The listing builds one solid part. Answer for the finished solid, in the listing's coordinates (mm). Face numbers are marked on the shaded views. A direction names the side the tool comes from. Give positions to 0.01 mm unless a question says otherwise; leave off trailing zeros. Write each loop counter-clockwise with the first axis right and the second up, starting at its lowest first coordinate (ties: lowest second). Pieces come first, ordered by that corner, then holes. Notation, with made-up numbers: (5, -7) -> (36, -7) arc R22 cw to (36, 23) -> close; hole circle Ø4 at (-13.75, -9.5). An arc over 180 degrees is marked (long way). One line per question, with ' | ' between items.
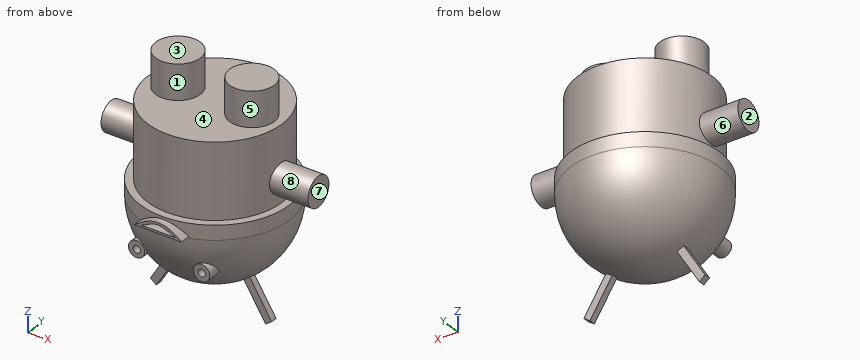
from build123d import *

# Parameters (mm, degrees)
F0_R          = 15
F3_DEPTH      = 30
F1_R          = 45
F4_DEPTH      = 50
F4_DEPTH_BACK = 6.5
F5_START      = -44
F2_R          = 50
F5_DEPTH      = 9.75
F6_R          = 10
F7_DEPTH      = 70
F8_R          = 10
F9_DEPTH      = 70
F12_R         = 5.5
F13_DEPTH     = 43.75
F14_R         = 2.5
F15_DEPTH     = 50.5
F17_DEPTH     = 4.25
F19_DEPTH     = 54.5
F21_DEPTH     = 63.5


with BuildPart() as f3:
    # F0 (on Top) → F3 (new body)
    with BuildSketch(Plane.XY):
        with Locations((-25, 0)):
            Circle(F0_R)
    extrude(amount=F3_DEPTH)



with BuildPart() as f3b:
    # F0 (on Top) → F3, piece 2 (new body)
    with BuildSketch(Plane.XY):
        with Locations((25, 0)):
            Circle(F0_R)
    extrude(amount=F3_DEPTH)


with BuildPart() as f3_1:
    add(f3.part)

    add(f3b.part)  # F4 merges F3b
    # F1 (on Top) → F4 (join, two sides)
    with BuildSketch(Plane.XY) as f4_sk:
        Circle(F1_R)
    extrude(amount=-F4_DEPTH)
    extrude(f4_sk.sketch, amount=F4_DEPTH_BACK)

    # F2 (on Top) → F5 (join)
    with BuildSketch(Plane.XY.offset(F5_START)):
        Circle(F2_R)
    extrude(amount=-F5_DEPTH)

    # F6 (on Right) → F7 (join)
    with BuildSketch(Plane.YZ):
        with Locations((0, -28)):
            Circle(F6_R)
    extrude(amount=F7_DEPTH)

    # F8 (on Right) → F9 (join)
    with BuildSketch(Plane.YZ):
        with Locations((0, -28)):
            Circle(F8_R)
    extrude(amount=-F9_DEPTH)

    # F10 (on Front) → F11 (revolve)
    with BuildSketch(Plane.XZ):
        with BuildLine():
            Line((0, -53.75), (0, -103.75))
            ThreePointArc((0, -103.75), (35.3553390593, -89.1053390593), (50, -53.75))
            Line((50, -53.75), (0, -53.75))
        make_face()
    revolve(axis=Axis((0, 0, -78.75), (0, 0, -1)))

    # F12 (on Front) → F13 (join)
    with BuildSketch(Plane.XZ):
        with Locations((22, -75.75)):
            Circle(F12_R)
        with Locations((-22, -75.75)):
            Circle(F12_R)
    extrude(amount=F13_DEPTH)

    # F14 (on Front) → F15 (cut)
    with BuildSketch(Plane.XZ):
        with Locations((22.0108069479, -75.75)):
            Circle(F14_R)
        with Locations((-21.8705814332, -75.75)):
            Circle(F14_R)
    extrude(amount=F15_DEPTH, mode=Mode.SUBTRACT)

    # F16 (on Front) → F17 (join)
    with BuildSketch(Plane.XZ):
        Polygon((37.273382177, -122.7384150805), (41.3573574255, -119.8537753855), (25.9457886256, -95.2878732623), (21.5874810644, -97.7384150805), align=None)
        Polygon((-40.6426425745, -120.3244923925), (-36.726617823, -123.4333105193), (-21.49733765, -98.4333105193), (-25.5781691914, -95.5442252089), align=None)
    extrude(amount=F17_DEPTH)

    # F18 (on Front) → F19 (join)
    with BuildSketch(Plane.XZ):
        with BuildLine():
            Line((-16, -52.6157000572), (16, -52.6157000572))
            add(Edge.make_bspline(
                [(16, -52.6157000572), (10.6081692502, -47.7225370705), (-0.6081692502, -43.4127992868), (-9.3918307498, -47.914664585), (-16, -52.6157000572)],
                knots=[0, 0, 0, 0, 0.5, 1, 1, 1, 1], degree=3))
        make_face()
    extrude(amount=F19_DEPTH)

    # F20 (on Front) → F21 (cut)
    with BuildSketch(Plane.XZ):
        with BuildLine():
            Line((-11, -51.2171401906), (12, -51.2171401906))
            add(Edge.make_bspline(
                [(12, -51.2171401906), (7.809161948, -49.4812574583), (-0.0193589542, -44.8915549483), (-7.190838052, -49.3467373151), (-11, -51.2171401906)],
                knots=[0, 0, 0, 0, 0.5096641908, 1, 1, 1, 1], degree=3))
        make_face()
    extrude(amount=F21_DEPTH, mode=Mode.SUBTRACT)


solid = f3_1.part
Item 1: Flat-ended cylindrical pins translate along their axes: pin 1 (12 mm diameter, centred on x = 16.5, y = 37, fed in from +Z); pin 2 (2.5 mm diameter, centred on x = -21.5, z = -76.5, fed in from -Y); pin 3 (1 mm diameter, centred on x = 6, z = -78.5, fed in from +Y). Find the tip coordinate at first contact, or state that the pin passes through.
Answers below:
pin 1: z = 6.5 | pin 2: y = 0 | pin 3: y = 43.32
Item 2: Find section A-A (x = 32). Write down the section's boundary in (y, z).
Answers below:
outline: (-38.42, -53.75) arc R38.42 ccw to (38.42, -53.75) -> (38.42, -44) -> (31.64, -44) -> (31.64, 6.5) -> (13.27, 6.5) -> (13.27, 30) -> (-13.27, 30) -> (-13.27, 6.5) -> (-31.64, 6.5) -> (-31.64, -44) -> (-38.42, -44) -> close; (-4.25, -114.33) -> (0, -114.33) -> (0, -104.94) -> (-4.25, -104.94) -> close
Item 3: Determine the mould class of the marked faces 1, 2, 3 and 4 for opening direction X: pulls with the +X half, pulls with the -X half, needs draft (parallel to the pull), parting line crosses it, or undercut.
Answers below:
face 1: undercut | face 2: pulls with the -X half | face 3: needs draft | face 4: undercut
Item 4: Consider line 1 (X direction, y = -22, z = -75.75); line 2 (X direction, y = -15, z = -75.75); line 3 (Y direction, x = -24, z = -46.5). Determine where each line is inside the solid, lowest interval first. Write a range as [from, to].
Answers below:
line 1: [-39.14, -24.37], [-19.37, 19.51], [24.51, 39.14] | line 2: [-42.32, -24.37], [-19.37, 19.51], [24.51, 42.32] | line 3: [-43.86, 43.86]
Item 5: Find section D-D (y = -30). Count the separate pieces of the cut face and the enclosed holes in it, then the cut area to 3 significant figures.
Answers below:
separate pieces: 1 | enclosed holes: 3 | area: 6,590 mm²
Item 6: A tool of negligible diameter and unlimited length cuts with its end or side. For the marked faces 5, 6, 7 and 8, from which of +Z, -Z, +X, -X, +Y, -Y can it reach the whole face along a straight path? Write none if from no direction.
Answers below:
face 5: +Z | face 6: -X | face 7: +Z, -Z, +X, +Y, -Y | face 8: +X
Item 7: Find section C-C (y = 4.5). Write down the section's boundary in (x, z).
Answers below:
outline: (-70, -36.93) -> (-44.77, -36.93) -> (-44.77, -44) -> (-49.8, -44) -> (-49.8, -53.75) arc R49.8 ccw to (49.8, -53.75) -> (49.8, -44) -> (44.77, -44) -> (44.77, -36.93) -> (70, -36.93) -> (70, -19.07) -> (44.77, -19.07) -> (44.77, 6.5) -> (39.31, 6.5) -> (39.31, 30) -> (10.69, 30) -> (10.69, 6.5) -> (-10.69, 6.5) -> (-10.69, 30) -> (-39.31, 30) -> (-39.31, 6.5) -> (-44.77, 6.5) -> (-44.77, -19.07) -> (-70, -19.07) -> close
Item 8: Find section B-B (z = -28). Write down the section's boundary in (x, y).
Answers below:
outline: (-70, -10) -> (-43.87, -10) arc R45 ccw to (43.87, -10) -> (70, -10) -> (70, 10) -> (43.87, 10) arc R45 ccw to (-43.87, 10) -> (-70, 10) -> close
